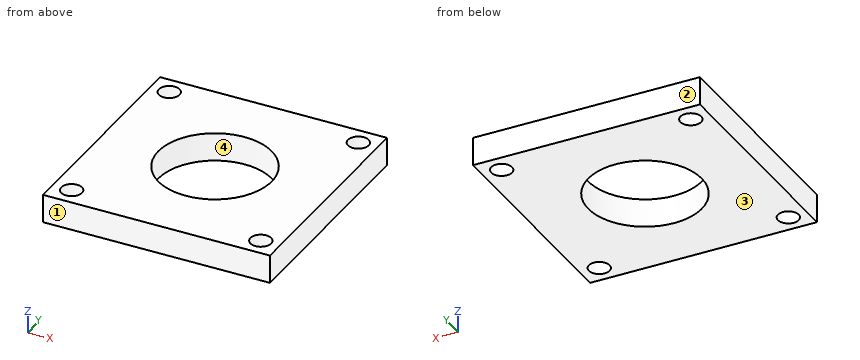
Autodesk Fusion 360 part; units mm, degrees
sketch "Sketch1" plane through (0, 0, 0) normal (0, 0, 1) x (1, 0, 0)
  line L0 (12, -12) -> (-12, -12)
  line L1 (-12, -12) -> (-12, 12)
  line L2 (-12, 12) -> (12, 12)
  line L3 (12, 12) -> (12, -12)
  line L4 (12, -12) -> (-12, 12) construction
  line L5 (-12, -12) -> (12, 12) construction
  dimension "d1" = 24
  dimension "d2" = 24
extrude "Extrude1" add sketch "Sketch1" along normal blind 3
sketch "Sketch2" plane through (0, 0, 3) normal (0, 0, 1) x (-1, 0, 0)
  line L0 (-12, -12) -> (12, -12)
  line L1 (12, -12) -> (12, 12)
  line L2 (12, 12) -> (-12, 12)
  line L3 (-12, 12) -> (-12, -12)
  circle A0 centre (10, -10) radius 1.1
  circle A1 centre (-10, -10) radius 1.1
  circle A2 centre (10, 10) radius 1.1
  circle A3 centre (-10, 10) radius 1.1
  dimension "d5" = 2.2
  dimension "d6" = 2.2
  dimension "d7" = 2.2
  dimension "d8" = 2.2
  dimension "d9" = 10
  dimension "d10" = 10
  dimension "d11" = 10
  dimension "d12" = 10
  dimension "d13" = 10
  dimension "d14" = 10
  dimension "d15" = 10
  dimension "d16" = 10
extrude "Extrude2" cut sketch "Sketch2" against normal through all contours A0 | A1 | A2 | A3
sketch "Sketch3" plane through (0, 0, 3) normal (0, 0, 1) x (-1, 0, 0)
  circle A0 centre (10, -10) radius 1.1
  circle A1 centre (10, 10) radius 1.1
  circle A2 centre (-10, -10) radius 1.1
  circle A3 centre (-10, 10) radius 1.1
  line L0 (-12, -12) -> (12, -12)
  line L1 (12, -12) -> (12, 12)
  line L2 (12, 12) -> (-12, 12)
  line L3 (-12, 12) -> (-12, -12)
  circle A4 centre (0, 0) radius 6
  dimension "d18" = 12
extrude "Extrude3" cut sketch "Sketch3" against normal blind 6 contours A4
Part model, mm, in its own coordinate system. Face numbers are marked on the shaded views. Round coordinates to 2 decimals unless told otherwise and drop trailing zeros. Write each loop counter-clockwise with the first axis right and the second up, starting at its lowest first coordinate (ties: lowest second). Pieces come first, ordered by that corner, then holes. Notation, with made-up numbers: M -16,29.25 L 38,29.25 A22 ccw 38,58.25 Z; hole C 51,69 d4. An arc over 180 degrees is marked long. Return JSON: item names as keys, results as strings. Group by question number.
(1) Saw through at C-C on z = 1.6. Write the cut outline in (x, y), then the cut area to 3 significant figures.
(2) Saw through at B-B on x = -10. Write the cut outline in (y, z), then the cut area to 3 significant figures.
(3) Saw through at A-A on y = 0. Write the cut outline in (x, z).
(4) Two-plate mould, pull along Y, no slides. Class the marked faces 1, 2, 3 and 4: +Y half, -Y half, draft (parallel to the pull), parting line (faces both ways), or undercut.
(5) Drill centre lines: probe 1 along X at (y, z) = (-10, 1.2); probe 2 along Y at (x, z) = (0, 1.2). Where is each one in solid material? Low to high.
Returned:
{
 "1": {"outline": "M -12,-12 L 12,-12 L 12,12 L -12,12 Z; hole C -10,-10 d2.2; hole C -10,10 d2.2; hole C 0,0 d12; hole C 10,-10 d2.2; hole C 10,10 d2.2", "area": "448 mm²"},
 "2": {"outline": "M -12,0 L -11.1,0 L -11.1,3 L -12,3 Z; M -8.9,0 L 8.9,0 L 8.9,3 L -8.9,3 Z; M 11.1,0 L 12,0 L 12,3 L 11.1,3 Z", "area": "58.8 mm²"},
 "3": {"outline": "M -12,0 L -6,0 L -6,3 L -12,3 Z; M 6,0 L 12,0 L 12,3 L 6,3 Z"},
 "4": {"face 1": "-Y half", "face 2": "+Y half", "face 3": "draft", "face 4": "undercut"},
 "5": {"probe 1": "-12 to -11.1, -8.9 to 8.9, 11.1 to 12", "probe 2": "-12 to -6, 6 to 12"}
}
